The model under review builds one solid part; all positions refer to its coordinate system, in mm. Face numbers are marked on the shaded views. Coordinates: 2 decimals unless noted, no trailing zeros. Write each loop counter-clockwise with the first axis right and the second up, starting at its lowest first coordinate (ties: lowest second). Pieces come first, ordered by that corner, then holes. Notation, with made-up numbers: (63.25, 43.25) - (81.25, 43.25) arc R17 cw to (81.25, 71.25) - close; hole circle Ø3 at (62, -2). An arc over 180 degrees is marked (long way). Return JSON: item names as keys, results as strings. Group by question number.
(1) We need section B-B on y = 41. State the section outline as (x, z) points.
(2) For pin 1 Ø4 at (x, z) = (-64, -1.5) entering from +Y; pin 2 Ø0.6 at (x, z) = (48, 1) entering from +Y; pin 3 Ø10 at (x, y) = (-39.5, -1) entering from +Z, all flat-tipped, find the tip position at first contact; note any pin that passes through.
(3) To check wall thickness, follow L1, parallel to X at y = -4, z = 3; L2, parallel to X at y = 48, z = 1.75; L3, parallel to X at y = -94.65, z = -0.55. State the ranges of each line that lie inside material, in increasing order. Write a range as from..to.
(4) Draft analysis for pull direction Y (two halves, no side actions). For the marked faces 1, 2 and 3, state which applies: released by +Y, released by -Y, zero draft, split by the parting line, or undercut.
(5) We need section C-C on y = -21.5. State the section outline as (x, z) points.
(6) We need section D-D on x = -60. State the section outline as (y, z) points, then the cut area to 3 significant figures.
(7) We need section A-A on x = 20. State the section outline as (y, z) points.
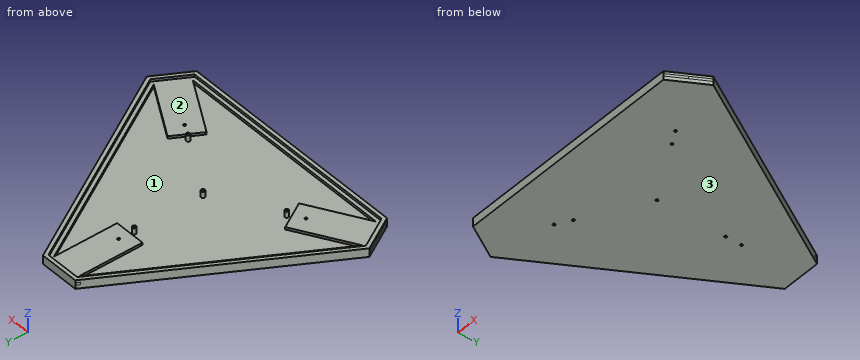
```python
from build123d import *

# Parameters (mm, degrees)
F0_R     = 1
F1_DEPTH = 2
F2_R     = 1
F3_DEPTH = 3
F4_R     = 1.5
F4_R_2   = 1
F5_DEPTH = 5
F7_DEPTH = 2


with BuildPart() as f1:
    # F0 (on Top) → F1 (new body)
    with BuildSketch(Plane.XY):
        Polygon((0, 52), (0, 0), (25, 0), (25, 52), (12.5, 52), align=None)
        with Locations((12.5, 9.3)):
            Circle(F0_R, mode=Mode.SUBTRACT)
        Polygon((109.4948452239, -116), (115.7448452239, -105.1746824527), (70.7115242271, -79.1746824527), (64.4615242271, -90), (58.2115242271, -100.8253175473), (103.2448452239, -126.8253175473), align=None)
        with Locations((72.5155604823, -94.65)):
            Circle(F0_R, mode=Mode.SUBTRACT)
        Polygon((-90.7448452239, -105.1746824527), (0, 52), (12.5, 52), (12.5, 58), (-3.4641016151, 58), (-5.1961524227, 55), (-50.5685750346, -23.5873412263), (-97.6730484541, -105.1746824527), (-89.6909976466, -119), (-84.4948452239, -116), align=None)
        Polygon((12.5, 52), (25, 52), (115.7448452239, -105.1746824527), (109.4948452239, -116), (114.6909976466, -119), (122.6730484541, -105.1746824527), (75.5685750346, -23.5873412263), (30.1961524227, 55), (28.4641016151, 58), (12.5, 58), align=None)
        Polygon((-45.7115242271, -79.1746824527), (-90.7448452239, -105.1746824527), (-84.4948452239, -116), (-78.2448452239, -126.8253175473), (-33.2115242271, -100.8253175473), (-39.4615242271, -90), align=None)
        with Locations((-47.5155604823, -94.65)):
            Circle(F0_R, mode=Mode.SUBTRACT)
        Polygon((-78.2448452239, -126.8253175473), (-84.4948452239, -116), (-89.6909976466, -119), (-81.708946839, -132.8253175473), (12.5, -132.8253175473), (106.708946839, -132.8253175473), (114.6909976466, -119), (109.4948452239, -116), (103.2448452239, -126.8253175473), align=None)
    extrude(amount=F1_DEPTH)

    # F2 (on face) → F3 (join)
    with BuildSketch(Plane(origin=(0, 0, 0), x_dir=(1, 0, 0), z_dir=(0, 0, -1))):
        Polygon((-3.4641016151, -58), (28.4641016151, -58), (122.6730484541, 105.1746824527), (106.708946839, 132.8253175473), (-81.708946839, 132.8253175473), (-97.6730484541, 105.1746824527), align=None)
        with Locations((12.5, -9.3)):
            Circle(F2_R, mode=Mode.SUBTRACT)
        Polygon((25, 0), (0, 0), (0, -52), (-90.7448452239, 105.1746824527), (-45.7115242271, 79.1746824527), (-33.2115242271, 100.8253175473), (-78.2448452239, 126.8253175473), (103.2448452239, 126.8253175473), (58.2115242271, 100.8253175473), (70.7115242271, 79.1746824527), (115.7448452239, 105.1746824527), (25, -52), align=None, mode=Mode.SUBTRACT)
        with Locations((-47.5155604823, 94.65)):
            Circle(F2_R, mode=Mode.SUBTRACT)
        with Locations((72.5155604823, 94.65)):
            Circle(F2_R, mode=Mode.SUBTRACT)
        Polygon((0, -52), (0, 0), (25, 0), (25, -52), (115.7448452239, 105.1746824527), (70.7115242271, 79.1746824527), (58.2115242271, 100.8253175473), (103.2448452239, 126.8253175473), (-78.2448452239, 126.8253175473), (-33.2115242271, 100.8253175473), (-45.7115242271, 79.1746824527), (-90.7448452239, 105.1746824527), align=None)
        with Locations((12.5, 3.64)):
            Circle(F2_R, mode=Mode.SUBTRACT)
        with Locations((12.5, 60)):
            Circle(F2_R, mode=Mode.SUBTRACT)
        with Locations((-36.3091917573, 88.18)):
            Circle(F2_R, mode=Mode.SUBTRACT)
        with Locations((61.3091917573, 88.18)):
            Circle(F2_R, mode=Mode.SUBTRACT)
    extrude(amount=F3_DEPTH)

    # F4 (on face) → F5 (join)
    with BuildSketch(Plane.XY):
        with Locations((-36.3091917573, -88.18)):
            Circle(F4_R)
        with Locations((-36.3091917573, -88.18)):
            Circle(F4_R_2, mode=Mode.SUBTRACT)
        with Locations((61.3091917573, -88.18)):
            Circle(F4_R)
        with Locations((61.3091917573, -88.18)):
            Circle(F4_R_2, mode=Mode.SUBTRACT)
        with Locations((12.5, -60)):
            Circle(F4_R)
        with Locations((12.5, -60)):
            Circle(F4_R_2, mode=Mode.SUBTRACT)
        with Locations((12.5, -3.64)):
            Circle(F4_R)
        with Locations((12.5, -3.64)):
            Circle(F4_R_2, mode=Mode.SUBTRACT)
    extrude(amount=F5_DEPTH)

    # F6 (on face) → F7 (join)
    with BuildSketch(Plane.XY.offset(2)):
        Polygon((106.708946839, -132.8253175473), (122.6730484541, -105.1746824527), (28.4641016151, 58), (-3.4641016151, 58), (-97.6730484541, -105.1746824527), (-81.708946839, -132.8253175473), align=None)
        Polygon((-94.208946839, -105.1746824527), (-47.9704988233, -25.0873412263), (-1.7320508076, 55), (12.5, 55), (26.7320508076, 55), (72.9704988233, -25.0873412263), (119.208946839, -105.1746824527), (112.0929214352, -117.5), (104.9768960314, -129.8253175473), (12.5, -129.8253175473), (-79.9768960314, -129.8253175473), (-87.0929214352, -117.5), align=None, mode=Mode.SUBTRACT)
    extrude(amount=F7_DEPTH)


solid = f1.part
```
Ans:
{
 "1": {"outline": "(-13.28, -3) - (38.28, -3) - (38.28, 4) - (34.81, 4) - (34.81, 2) - (31.35, 2) - (31.35, 0) - (25, 0) - (25, 2) - (0, 2) - (0, 0) - (-6.35, 0) - (-6.35, 2) - (-9.81, 2) - (-9.81, 4) - (-13.28, 4) - close"},
 "2": {"pin 1": "y = -43.39", "pin 2": "y = 24.68", "pin 3": "z = 4"},
 "3": {"L1": "-39.26..-35.8, 11.04..11.57, 13.43..13.96, 60.8..64.26", "L2": "-9.24..-2.31, 0..25, 27.31..34.24", "L3": "-91.6..-48.52, -46.52..71.52, 73.52..116.6"},
 "4": {"face 1": "undercut", "face 2": "undercut", "face 3": "zero draft"},
 "5": {"outline": "(-49.36, -3) - (74.36, -3) - (74.36, 4) - (70.9, 4) - (70.9, 2) - (67.44, 2) - (67.44, 0) - (-42.44, 0) - (-42.44, 2) - (-45.9, 2) - (-45.9, 4) - (-49.36, 4) - close"},
 "6": {"outline": "(-132.83, -3) - (-39.92, -3) - (-39.92, 4) - (-45.92, 4) - (-45.92, 2) - (-51.92, 2) - (-51.92, 0) - (-87.42, 0) - (-87.42, 2) - (-116.29, 2) - (-116.29, 0) - (-126.83, 0) - (-126.83, 2) - (-129.83, 2) - (-129.83, 4) - (-132.83, 4) - close", "area": "390 mm²"},
 "7": {"outline": "(-132.83, -3) - (58, -3) - (58, 4) - (55, 4) - (55, 2) - (0, 2) - (0, 0) - (-126.83, 0) - (-126.83, 2) - (-129.83, 2) - (-129.83, 4) - (-132.83, 4) - close"}
}
